Could you check a few things on this drawing? It's one solid part, dimensions in mm from its lowest x, y, z. Give positions to 0.01 mm unless a question says otherwise; leave off trailing zeros. Order: outer loops, then holes, each group sorted by start corner. A loop starts at its lowest first (then second) coordinate and runs counter-clockwise, first axis right, second up.
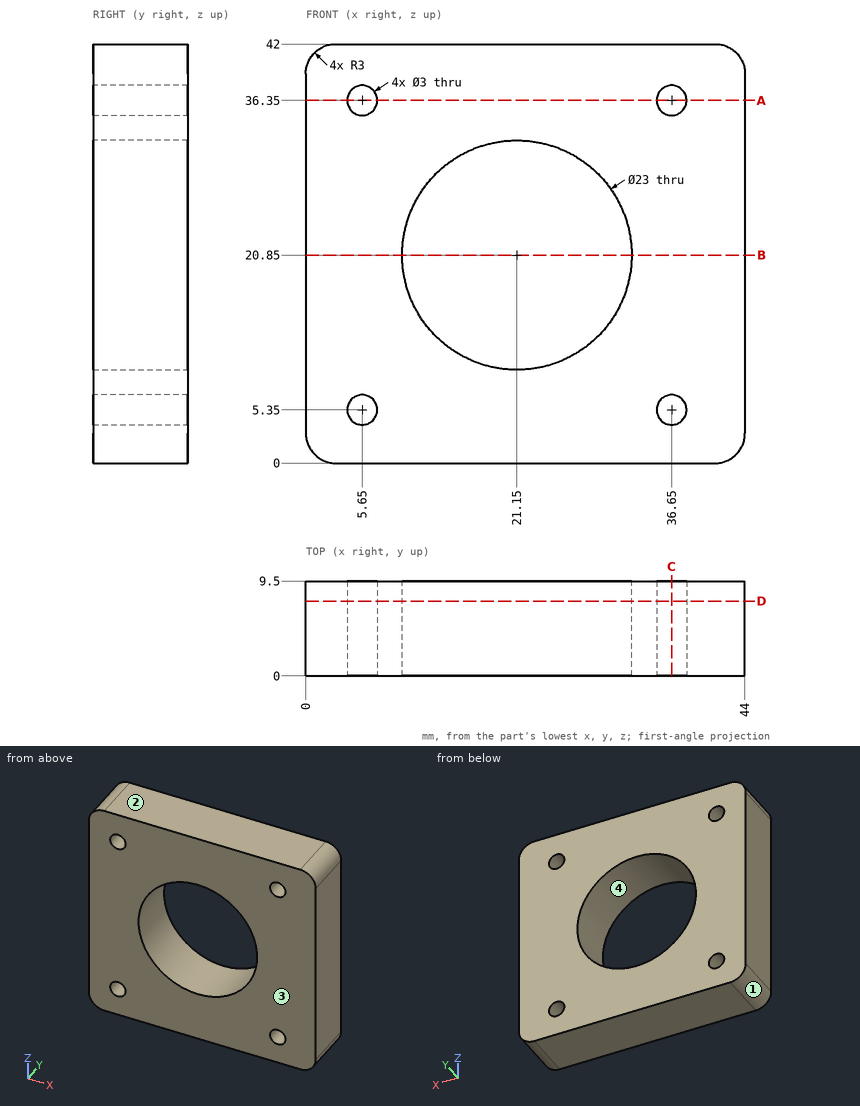
Q1. If we section it at B-B on z = 20.85: List the corners of the cut face in (x, y) for me, plus the area to 4 significant figures.
Filled sheet:
outline: (0, 0) - (9.65, 0) - (9.65, 9.5) - (0, 9.5) - close; (32.65, 0) - (44, 0) - (44, 9.5) - (32.65, 9.5) - close
area: 199.5 mm2
Q2. If we section it at C-C on x = 36.65: List the corners of the cut face in (y, z) for me, plus the area to 3 significant figures.
Filled sheet:
outline: (0, 0) - (9.5, 0) - (9.5, 3.85) - (0, 3.85) - close; (0, 6.85) - (9.5, 6.85) - (9.5, 34.85) - (0, 34.85) - close; (0, 37.85) - (9.5, 37.85) - (9.5, 42) - (0, 42) - close
area: 342 mm2
Q3. I need wall thicknesses on L1, parallel to X at y = 6.75, z = 36.35; L2, parallel to Z at x = 18.5, y = 5; L3, parallel to X at y = 2.5, z = 14.5. Which ranges of each line are inside material? Lowest first, please.
Filled sheet:
L1: x = 0 to 4.15, 7.15 to 35.15, 38.15 to 44
L2: z = 0 to 9.66, 32.04 to 42
L3: x = 0 to 11.56, 30.74 to 44
Q4. I'm going to push a flat-ended pin straight in: P1, Ø2.5, axis at x = 36.65, z = 5.35, coming from the -Y side. Where does the tip first touch, or does it pass through?
Filled sheet:
P1: passes through
Q5. If we section it at A-A on z = 36.35: List the corners of the cut face in (x, y) for me, plus the area to 3 significant figures.
Filled sheet:
outline: (0, 0) - (4.15, 0) - (4.15, 9.5) - (0, 9.5) - close; (7.15, 0) - (35.15, 0) - (35.15, 9.5) - (7.15, 9.5) - close; (38.15, 0) - (44, 0) - (44, 9.5) - (38.15, 9.5) - close
area: 361 mm2
Q6. If we section it at D-D on y = 7.5: List the corners of the cut face in (x, z) for me.
Filled sheet:
outline: (0, 3) arc R3 ccw to (3, 0) - (41, 0) arc R3 ccw to (44, 3) - (44, 39) arc R3 ccw to (41, 42) - (3, 42) arc R3 ccw to (0, 39) - close; hole circle Ø3 at (5.65, 5.35); hole circle Ø3 at (5.65, 36.35); hole circle Ø23 at (21.15, 20.85); hole circle Ø3 at (36.65, 5.35); hole circle Ø3 at (36.65, 36.35)
Q7. Thinking about a two-plate mould opening in Z: for the marked faces 1, 2, 3 and 4, which applies, released by +Z, released by -Z, zero draft, split by the parting line, or undercut?
Filled sheet:
face 1: released by -Z
face 2: released by +Z
face 3: zero draft
face 4: undercut
